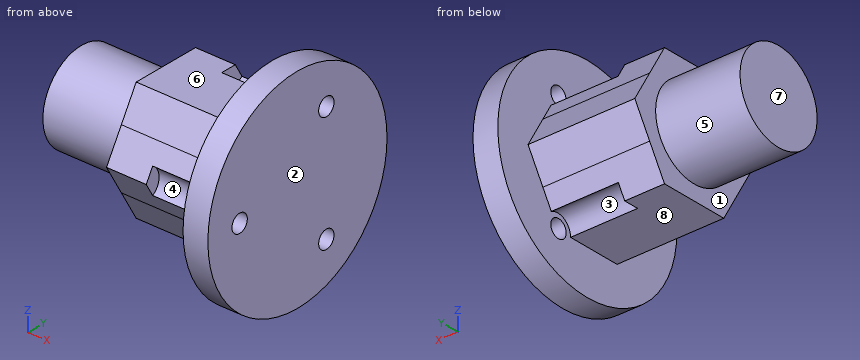
Autodesk Inventor part; units mm, degrees
ref_plane "YZ Plane" through (0, 0, 0) normal (1, 0, 0) x (0, 1, 0)
ref_plane "XZ Plane" through (0, 0, 0) normal (0, 1, 0) x (-1, 0, 0)
ref_plane "XY Plane" through (0, 0, 0) normal (0, 0, 1) x (1, 0, 0)
sketch "Sketch1" plane through (0, 0, 0) normal (0, 0, 1) x (1, 0, 0)
  line L0 (0, 0) -> (-13, 0)
  line L1 (-13, 0) -> (-13, 9)
  line L2 (-13, 9) -> (0, 9)
  line L3 (0, 9) -> (0, 12)
  line L4 (0, 12) -> (8, 12)
  line L5 (8, 12) -> (8, 11)
  line L6 (33, 0) -> (0, 0)
  line L7 (8, 11) -> (8, 0)
  dimension "d0" = 13
  dimension "d1" = 9
  dimension "d2" = 13
  dimension "d3" = 3
  dimension "d4" = 8
  dimension "d5" = 1
sketch "Sketch1 outline for Revolution1" plane through (0, 0, 0) normal (0, 0, 1) x (1, 0, 0)
  line L0 (8, 11) -> (8, 12)
  line L1 (8, 0) -> (8, 11)
  line L2 (0, 0) -> (8, 0)
  line L3 (-13, 0) -> (0, 0)
  line L4 (-13, 9) -> (-13, 0)
  line L5 (0, 9) -> (-13, 9)
  line L6 (0, 12) -> (0, 9)
  line L7 (8, 12) -> (0, 12)
revolve "Revolution1" add sketch "Sketch1 outline for Revolution1" angle 360 about axis through (33, 0, 0) along (-1, 0, 0)
sketch "Sketch2" plane through (8, 0, 0) normal (1, 0, 0) x (0, 0, -1)
  circle A0 centre (0, 0) radius 12
  line L0 (12, -6.928203) -> (0, -13.856406)
  line L1 (0, -13.856406) -> (-12, -6.928203)
  line L2 (-12, -6.928203) -> (-12, 6.928203)
  line L3 (-12, 6.928203) -> (0, 13.856406)
  line L4 (0, 13.856406) -> (12, 6.928203)
  line L5 (12, 6.928203) -> (12, -6.928203)
  circle A1 centre (0, 0) radius 11
  point P0 (0, 0)
  point P1 (12, 0)
  point P2 (6, 10.392305)
  point P3 (6, -10.392305)
  point P4 (-6, 10.392305)
  point P5 (-12, 0)
  point P6 (-6, -10.392305)
  dimension "d12" = 24
  dimension "d13" = 0
sketch "Sketch2 outline for Extrusion1" plane through (8, 0, 0) normal (1, 0, 0) x (0, 0, -1)
  line L0 (12, 0) -> (12, 6.928203)
  arc A0 (6, 10.392305) -> (12, 0) centre (0, 0) cw
  line L1 (12, 6.928203) -> (6, 10.392305)
  line L2 (12, -6.928203) -> (12, 0)
  line L3 (6, -10.392305) -> (12, -6.928203)
  arc A1 (12, 0) -> (6, -10.392305) centre (0, 0) cw
  line L4 (6, 10.392305) -> (0, 13.856406)
  arc A2 (-6, 10.392305) -> (6, 10.392305) centre (0, 0) cw
  line L5 (0, 13.856406) -> (-6, 10.392305)
  line L6 (-6, 10.392305) -> (-12, 6.928203)
  arc A3 (-12, 0) -> (-6, 10.392305) centre (0, 0) cw
  line L7 (-12, 6.928203) -> (-12, 0)
  line L8 (-12, 0) -> (-12, -6.928203)
  arc A4 (-6, -10.392305) -> (-12, 0) centre (0, 0) cw
  line L9 (-12, -6.928203) -> (-6, -10.392305)
  line L10 (-6, -10.392305) -> (0, -13.856406)
  arc A5 (6, -10.392305) -> (-6, -10.392305) centre (0, 0) cw
  line L11 (0, -13.856406) -> (6, -10.392305)
extrude "Extrusion1" add sketch "Sketch2 outline for Extrusion1" against normal blind 8 contours A0 L1 L0 | L2 L3 A1 | A2 L5 L4 | L11 L10 A5 | A3 L7 L6 | L9 L8 A4
sketch "Sketch3" plane through (-13, 0, 0) normal (-1, 0, 0) x (0, 0, 1)
  circle A0 centre (0, 0) radius 7.75
  circle A1 centre (0, 0) radius 6.5
  point P0 (0, 0)
  dimension "d18" = 13
sketch "Sketch3 outline for Extrusion2" plane through (-13, 0, 0) normal (-1, 0, 0) x (0, 0, 1)
  circle A0 centre (0, 0) radius 6.5
extrude "Extrusion2" cut sketch "Sketch3 outline for Extrusion2" against normal blind 13
sketch "Sketch4" plane through (0, 0, 0) normal (-1, 0, 0) x (0, 0, 1)
  circle A0 centre (0, 0) radius 1.55
  point P0 (0, 0)
  dimension "d21" = 3.1
sketch "Sketch4 outline for Extrusion3" plane through (0, 0, 0) normal (-1, 0, 0) x (0, 0, 1)
  circle A0 centre (0, 0) radius 1.55
extrude "Extrusion3" cut sketch "Sketch4 outline for Extrusion3" against normal through all
ref_plane "작업 평면2" through (20.5, 0, -6) normal (0, 0, 1) x (1, 0, 0)
sketch "스케치7" plane through (20.5, 0, -6) normal (0, 0, 1) x (1, 0, 0)
  circle A0 centre (6.75, 0) radius 1.3
  line L0 (6.75, -3.175426) -> (4, -1.587713)
  line L1 (4, -1.587713) -> (4, 1.587713)
  line L2 (4, 1.587713) -> (6.75, 3.175426)
  line L3 (6.75, 3.175426) -> (9.5, 1.587713)
  line L4 (9.5, 1.587713) -> (9.5, -1.587713)
  line L5 (9.5, -1.587713) -> (6.75, -3.175426)
  line L6 (12.5, 6) -> (12.5, -6)
  point P0 (-20.5, 0)
  point P1 (9.5, 0)
  dimension "d27" = 2.6
  dimension "d28" = 5.5
  dimension "d37" = 3
extrude "돌출6" [suppressed]
extrude "돌출7" [suppressed]
sketch "스케치8" plane through (33, 0, 0) normal (1, 0, 0) x (0, 0, -1)
  point P0 (0, 0)
sketch "스케치9" plane through (8, -6.928203, 12) normal (1, 0, 0) x (0, 0, -1)
  circle A0 centre (12, 6.928203) radius 16
  dimension "d38" = 32
extrude "돌출8" [suppressed]
move faces "이동1" translate (12.5, 0, 10) faces at (8, 7.353412, -4.2935)
sketch "스케치10" plane through (20.5, -6.928203, 12) normal (1, 0, 0) x (0, 0, -1)
  circle A0 centre (12, 6.928203) radius 1.55
  circle A1 centre (12, 6.928203) radius 25
  dimension "d44" = 50
extrude "돌출9" [suppressed]
sketch "스케치11" plane through (20.5, 0, 0) normal (-1, 0, 0) x (0, 0, 1)
  circle A0 centre (0, 0) radius 1.55
  circle A1 centre (0, 0) radius 15
  circle A2 centre (0, 0) radius 16
  point P0 (0, 0)
  dimension "d49" = 30
  dimension "d50" = 32
extrude "돌출10" [suppressed]
sketch "스케치12" plane through (20.5, -6.928203, 12) normal (1, 0, 0) x (0, 0, -1)
  circle A0 centre (12, 6.928203) radius 20.916385
sketch "스케치12 outline for 돌출11" plane through (20.5, -6.928203, 12) normal (1, 0, 0) x (0, 0, -1)
  circle A0 centre (12, 6.928203) radius 20.916385
extrude "돌출11" add sketch "스케치12 outline for 돌출11" along normal blind 10
sketch "스케치14" plane through (30.5, 0, 0) normal (1, 0, 0) x (0, 0, -1)
  circle A0 centre (0, 0) radius 13.5
  circle A1 centre (0, -13.5) radius 1.795072
  circle A2 centre (11.691343, 6.75) radius 1.795072
  circle A3 centre (-11.691343, 6.75) radius 1.795072
  dimension "d59" = 27
  dimension "d64" = 360
sketch "스케치14 outline for 돌출13" plane through (30.5, 0, 0) normal (1, 0, 0) x (0, 0, -1)
  circle A0 centre (0, -13.5) radius 1.795072
  circle A1 centre (11.691343, 6.75) radius 1.795072
  circle A2 centre (-11.691343, 6.75) radius 1.795072
extrude "돌출13" cut sketch "스케치14 outline for 돌출13" against normal blind 15
sketch "스케치15" plane through (30.5, 0, 0) normal (1, 0, 0) x (0, 0, -1)
  point P0 (0, 0)
sketch "스케치16" plane through (20.5, 0, 0) normal (-1, 0, 0) x (0, 0, 1)
  circle A0 centre (0, -13.856406) radius 3
  circle A1 centre (11.691343, 6.75) radius 1.795072
  circle A2 centre (11.691343, 6.75) radius 3
  circle A3 centre (-12, 6.928203) radius 3
  point P0 (0, 0)
  dimension "d66" = 6
  dimension "d67" = 6
  dimension "d68" = 6
sketch "스케치16 outline for 돌출14" plane through (20.5, 0, 0) normal (-1, 0, 0) x (0, 0, 1)
  circle A0 centre (11.691343, 6.75) radius 3
  circle A1 centre (-12, 6.928203) radius 3
  circle A2 centre (0, -13.856406) radius 3
extrude "돌출14" cut sketch "스케치16 outline for 돌출14" along normal blind 11.499
move faces "이동2" translate (-3, 0, 0) faces at (30.5, 0.037854, 0.072124)
move faces "이동3" translate (9, 0, 0) faces at (0, 0.36161, -10.978127)
move faces "이동4" translate (5, 0, 0) faces at (-13, 8.063695, 0.97911)
move faces "이동5" translate (-8, 0, 0) faces at (9, -0.36161, -10.978127)
move faces "이동6" translate (-25.75, 0, 0) faces at (13.666667, -0.124723, 1.544974)
move faces "이동7" translate (-8, 0, 0) faces at (-8, 8.063695, 0.97911)
move faces "이동8" translate (-36.5, 0, 0) faces at (20.5, -0.007186, -0.457486)
move faces "이동9" translate (-16, 0, 0) faces at (0, -0.518517, 4.787041)
move faces "이동10" translate (2, 0, 0) faces at (20.5, -1, -14.972128)
properties part number "HEX HUB_Version2 (cheeta)"
Work out the finished part from the listing and answer in its coordinate system (mm). Face numbers are marked on the shaded views. A direction names the side the tool comes from. Give positions to 0.01 mm unless a question says otherwise; leave off trailing zeros. Loops run counter-clockwise (first coordinate to the right, second up) from the corner with the lowest first, then second, coordinate; pieces in that order, holes last. Notation, with made-up numbers: (4.5, 13) - (63.5, 13) arc R16 cw to (63.5, 21) - close; hole circle Ø6 at (-38.5, -32.5). An arc over 180 degrees is marked (long way). Answer in a Markdown table with one row per item. Add a question column.
Q1. Determine the mould class of the marked faces 1, 2 and 3 for opening direction X: released by +X, released by -X, zero draft, split by the parting line, or undercut.
Q2. Each of these flat-tipped pins is pushed along its axis until it touches: P1, Ø4, axis at x = -7, z = 9.5, coming from the -Y side; P2, Ø7, axis at x = 16.5, y = 3, coming from the +Z side; P3, Ø1.5, axis at x = -0.5, y = 4.5, coming from the +Z side. Where does it stop, or does it pass through?
Q3. The part is cut by section C-C (x = 17.5). Determine the outline of the cut face in (y, z), and give its area (3 significant figures).
Q4. The part is cut by section B-B (x = 24.5). Determine the outline of the cut face in (y, z).
Q5. A tool of negligible diameter and unlimited length cuts with its end or side. For the marked faces 4, 5, 6, 7 and 8, from which of +Z, -Z, +X, -X, +Y, -Y can it reach the whole face along a straight path? Write none if from no direction.
Q6. The part is cut by section A-A (y = 0). Determine the outline of the cut face in (x, z), and give its area (3 significant figures).
Q7. The part is cut by section D-D (z = 17). Determine the outline of the cut face in (x, y), and give its area (3 significant figures).
Q8. Consider line 1 along Z through (x, y) = (23, 6); line 2 along X through (y, z) = (11, -3); line 3 along X through (y, z) = (12.5, 13). Determine where each line is inside the solid, lowest interval first.
Solution:
| question | item | result |
|---|---|---|
| 1 | face 1 | released by -X |
| 1 | face 2 | released by +X |
| 1 | face 3 | undercut |
| 2 | P1 | stops at y = -4.97 |
| 2 | P2 | stops at z = 12 |
| 2 | P3 | stops at z = 8.18 |
| 3 | outline | (-12.36, -2.6) - (-10.39, -6) - (-6.93, -12) - (3.93, -12) arc R3 cw to (8.43, -9.4) - (10.39, -6) - (13.86, 0) - (10.39, 6) - (8.51, 9.26) arc R3 cw to (3.77, 12) - (-6.93, 12) - (-10.39, 6) - (-12.36, 2.6) arc R3 cw to start |
| 3 | area | 469 mm² |
| 4 | outline | circle Ø41.83 at (0, 0); hole circle Ø3.59 at (-13.5, 0); hole circle Ø3.59 at (6.75, -11.69); hole circle Ø3.59 at (6.75, 11.69) |
| 5 | face 4 | -Y |
| 5 | face 5 | -X |
| 5 | face 6 | +Z, -X, +Y, -Y |
| 5 | face 7 | +Z, -Z, -X, +Y, -Y |
| 5 | face 8 | -Z, -X, +Y, -Y |
| 6 | outline | (-16, -9) - (1, -9) - (1, -12) - (22.5, -12) - (22.5, -20.92) - (27.5, -20.92) - (27.5, 20.92) - (22.5, 20.92) - (22.5, 12) - (1, 12) - (1, 9) - (-16, 9) - close |
| 6 | area | 1,030 mm² |
| 7 | outline | (22.5, -12.19) - (27.5, -12.19) - (27.5, 12.19) - (22.5, 12.19) - close |
| 7 | area | 122 mm² |
| 8 | line 1 | z = -20.04 to -13.32, -10.06 to 10.06, 13.32 to 20.04 |
| 8 | line 2 | x = 1 to 27.5 |
| 8 | line 3 | x = 22.5 to 27.5 |
